```python
from build123d import *

# Parameters (mm, degrees)
ESQUISSE1_W             = 40
ESQUISSE1_H             = 18
BOSS_EXTRU_1_DEPTH      = 12
ESQUISSE2_W             = 40
ESQUISSE2_H             = 12
BOSS_EXTRU_2_DEPTH      = 10
ENL_V_MAT_EXTRU_1_DEPTH = 12
ESQUISSE4_R             = 2.5
ENL_V_MAT_EXTRU_2_DEPTH = 28
ESQUISSE5_R             = 2.5
ENL_V_MAT_EXTRU_3_DEPTH = 12
ESQUISSE7_R             = 3.5
ENL_V_MAT_EXTRU_4_DEPTH = 4
ESQUISSE6_R             = 3.5
ENL_V_MAT_EXTRU_5_DEPTH = 12
CONG_1_R                = 2
ESQUISSE8_W             = 63.620200945
ESQUISSE8_H             = 32.659215008
ENL_V_MAT_EXTRU_6_DEPTH = 12
CONG_3_R                = 2
ENL_V_MAT_EXTRU_7_DEPTH = 4


with BuildPart() as part:
    # Esquisse1 → Boss.-Extru.1 (new body)
    with BuildSketch(Plane.XY):
        with Locations((3.185612757, 0.725848564)):
            Rectangle(ESQUISSE1_W, ESQUISSE1_H)
    extrude(amount=BOSS_EXTRU_1_DEPTH)

    # Esquisse2 → Boss.-Extru.2 (add)
    with BuildSketch(Plane.XZ.offset(8.274151436)):
        with Locations((3.185612757, 6)):
            Rectangle(ESQUISSE2_W, ESQUISSE2_H)
    extrude(amount=BOSS_EXTRU_2_DEPTH)

    # Esquisse3 → Enlèv. mat.-Extru.1 (cut)
    with BuildSketch(Plane.XY.offset(12)):
        with BuildLine():
            Line((-2.864387243, -18.274151436), (9.235612757, -18.274151436))
            ThreePointArc((9.235612757, -18.274151436), (3.185612757, -12.224151436), (-2.864387243, -18.274151436))
        make_face()
    extrude(amount=-ENL_V_MAT_EXTRU_1_DEPTH, mode=Mode.SUBTRACT)

    # Esquisse4 → Enlèv. mat.-Extru.2 (cut)
    with BuildSketch(Plane.XZ.offset(18.274151436)):
        with Locations(Location((-9.839387243, 6, 0), (0, 0, 270))):
            Circle(ESQUISSE4_R)
        with Locations(Location((16.210612757, 6, 0), (0, 0, 270))):
            Circle(ESQUISSE4_R)
    extrude(amount=-ENL_V_MAT_EXTRU_2_DEPTH, mode=Mode.SUBTRACT)

    # Esquisse5 → Enlèv. mat.-Extru.3 (cut)
    with BuildSketch(Plane.XY.offset(12)):
        with Locations((9.185612757, 0.725848564)):
            Circle(ESQUISSE5_R)
        with Locations((-2.814387243, 0.725848564)):
            Circle(ESQUISSE5_R)
    extrude(amount=-ENL_V_MAT_EXTRU_3_DEPTH, mode=Mode.SUBTRACT)

    # Esquisse7 → Enlèv. mat.-Extru.4 (cut)
    with BuildSketch(Plane(origin=(0, 0, 0), x_dir=(-1, 0, 0), z_dir=(0, 0, -1))):
        with Locations((-9.185612757, 0.725848564)):
            Circle(ESQUISSE7_R)
        with Locations((2.814387243, 0.725848564)):
            Circle(ESQUISSE7_R)
    extrude(amount=-ENL_V_MAT_EXTRU_4_DEPTH, mode=Mode.SUBTRACT)

    # Esquisse6 → Enlèv. mat.-Extru.5 (cut)
    with BuildSketch(Plane(origin=(0, 9.725848564, 0), x_dir=(1, 0, 0), z_dir=(0, 1, 0))):
        with Locations(Location((16.210612757, -6, 0), (0, 0, 270))):
            Circle(ESQUISSE6_R)
        with Locations(Location((-9.839387243, -6, 0), (0, 0, 270))):
            Circle(ESQUISSE6_R)
    extrude(amount=-ENL_V_MAT_EXTRU_5_DEPTH, mode=Mode.SUBTRACT)

    # Congé1
    cong_1_edges = [part.edges().sort_by_distance(p)[0] for p in [
        (3.185612757, 9.725848564, 0),
        (23.185612757, -4.274151436, 0),
        (-16.814387243, -4.274151436, 0),
        (-16.814387243, 9.725848564, 6),
        (23.185612757, 9.725848564, 6),
    ]]
    fillet(cong_1_edges, radius=CONG_1_R)

    # Esquisse8 → Enlèv. mat.-Extru.6 (cut)
    with BuildSketch(Plane(origin=(0, 0, 0), x_dir=(-1, 0, 0), z_dir=(0, 0, -1))):
        with Locations((-6.809355957, 9.055456068)):
            Rectangle(ESQUISSE8_W, ESQUISSE8_H)
    extrude(amount=-ENL_V_MAT_EXTRU_6_DEPTH, mode=Mode.SUBTRACT)

    # Congé3
    cong_3_edges = [part.edges().sort_by_distance(p)[0] for p in [
        (-16.228600805, -7.274151436, 0.585786438),
        (23.185612757, -7.274151436, 7),
        (-16.814387243, -7.274151436, 7),
        (22.59982632, -7.274151436, 0.585786438),
        (3.185612757, -7.274151436, 0),
    ]]
    fillet(cong_3_edges, radius=CONG_3_R)

    # Esquisse9 → Enlèv. mat.-Extru.7 (cut)
    with BuildSketch(Plane(origin=(0, -7.274151436, 0), x_dir=(1, 0, 0), z_dir=(0, 1, 0))):
        Polygon((-5.509260224, -6), (-7.674323733, -2.25), (-12.004450752, -2.25), (-14.169514261, -6), (-12.004450752, -9.75), (-7.674323733, -9.75), align=None)
        Polygon((11.880485739, -6), (14.045549248, -9.75), (18.375676267, -9.75), (20.540739776, -6), (18.375676267, -2.25), (14.045549248, -2.25), align=None)
    extrude(amount=-ENL_V_MAT_EXTRU_7_DEPTH, mode=Mode.SUBTRACT)


solid = part.part
```
For this review, take the finished solid that the model builds, in its own axes (mm). A direction names the side the tool comes from. Coordinates: 2 decimals unless noted, no trailing zeros. Loops run counter-clockwise (first coordinate to the right, second up) from the corner with the lowest first, then second, coordinate; pieces in that order, holes last.
1. For line 1 (X direction, y = -17, z = 6); line 2 (X direction, y = -13.25, z = 6); line 3 (Y direction, x = 12.5, z = 6), list the stretches that pass through material, from the lowest coordinate up.
2. For faces 4 (the flat face through (-10, -9, 2.25)), 5 (the flat face through (3, -12, 0)), list the 3-axis set-ups (+Z, -Z, +X, -X, +Y, -Y) from which the entire face can be reached by the end or side of a thin tool; tool diameter is ignored.
3. Mouldability with a two-part tool opening along Z and no side actions: class faces 1 (the flat face through (16, -9, 9.75)), 2 (the cylindrical face through (-16.24, -13.84, 0.6)), 3 (the flat face through (23.186, -14, 7)) as +Z half, -Z half, draft (parallel to the pull), parting line (faces both ways), or undercut.
4. Add section C-C, the plane x = 0.5. Give the boundary of the cut face in (y, z).
5. Add section B-B, the plane z = 5.5. Give the boundary of the cut face in (x, y).
6. Add section D-D, the plane y = -8.75. Give the boundary of the cut face in (x, z).
7. Insertion check: P1, Ø6.5, axis at x = 16.21, z = 6, coming from the +Y side; P2, Ø1.5, axis at x = 4.5, z = 9, coming from the -Y side. Each pin has a flat end and moves straight along its axis. Give the tip position at first contact, or say it passes through.
8. Add section A-A, the plane y = -13.5. Give the boundary of the cut face in (x, z), then the cut area to 3 significant figures.
Result:
1. line 1: x = -16.81 to -12.34, -7.34 to -2.73, 9.1 to 13.71, 18.71 to 23.19
1. line 2: x = -16.81 to -12.34, -7.34 to -0.18, 6.56 to 13.71, 18.71 to 23.19
1. line 3: y = -18.27 to -11.27
2. face 4: +Y
2. face 5: -Z, +X, -X, +Y, -Y
3. face 1: undercut
3. face 2: -Z half
3. face 3: draft
4. outline: (-12.85, 0) - (-9.27, 0) arc R2 ccw to (-7.27, 2) - (-7.27, 12) - (-12.85, 12) - close
5. outline: (-16.81, -18.27) - (-12.29, -18.27) - (-12.29, -11.27) - (-13.88, -11.27) - (-13.88, -7.27) - (-14.81, -7.27) arc R2 ccw to (-16.81, -9.27) - close; (-7.39, -18.27) - (-2.86, -18.27) arc R6.05 cw to (9.24, -18.27) - (13.76, -18.27) - (13.76, -11.27) - (12.17, -11.27) - (12.17, -7.27) - (-5.8, -7.27) - (-5.8, -11.27) - (-7.39, -11.27) - close; (18.66, -18.27) - (23.19, -18.27) - (23.19, -9.27) arc R2 ccw to (21.19, -7.27) - (20.25, -7.27) - (20.25, -11.27) - (18.66, -11.27) - close
6. outline: (-16.74, 2) arc R1.93 ccw to (-14.81, 0.07) - (21.19, 0.07) arc R1.93 ccw to (23.12, 2) - (23.12, 12) - (-16.74, 12) - close; hole (-14.17, 6) - (-12, 2.25) - (-7.67, 2.25) - (-5.51, 6) - (-7.67, 9.75) - (-12, 9.75) - close; hole (11.88, 6) - (14.05, 2.25) - (18.38, 2.25) - (20.54, 6) - (18.38, 9.75) - (14.05, 9.75) - close
7. P1: stops at y = -11.27
7. P2: stops at y = -12.59
8. outline: (-16.81, 2) arc R2 ccw to (-14.81, 0) - (-0.53, 0) - (-0.53, 12) - (-16.81, 12) - close; (6.9, 0) - (21.19, 0) arc R2 ccw to (23.19, 2) - (23.19, 12) - (6.9, 12) - close; hole circle Ø5 at (-9.84, 6); hole circle Ø5 at (16.21, 6)
8. area: 350 mm2
